```python
from build123d import *

# Parameters (mm, degrees)
F0_W     = 85
F0_H     = 19.05
F0_R     = 1.6
F0_R_2   = 4.75
F1_DEPTH = 6.35
F2_R     = 1.5
F3_DEPTH = 5
F4_R     = 3


with BuildPart() as f1:
    # F0 (on Front) → F1 (new body)
    with BuildSketch(Plane.XZ):
        Rectangle(F0_W, F0_H)
        with Locations((-15.5, 0)):
            Circle(F0_R, mode=Mode.SUBTRACT)
        with Locations((32.5, 0)):
            Circle(F0_R_2, mode=Mode.SUBTRACT)
    extrude(amount=F1_DEPTH)

    # F2 (on face) → F3 (cut)
    with BuildSketch(Plane(origin=(0, 0, -9.525), x_dir=(1, 0, 0), z_dir=(0, 0, -1))):
        with Locations((-25.5, 3.175)):
            Circle(F2_R)
        with Locations((25.5, 3.175)):
            Circle(F2_R)
    extrude(amount=-F3_DEPTH, mode=Mode.SUBTRACT)

    # F4
    f4_edges = [f1.edges().sort_by_distance(p)[0] for p in [
        (-42.5, -3.175, -9.525),
        (42.5, -3.175, -9.525),
        (42.5, -3.175, 9.525),
        (-42.5, -3.175, 9.525),
    ]]
    fillet(f4_edges, radius=F4_R)


solid = f1.part
```
The listing builds one solid part. Answer for the finished solid, in the listing's coordinates (mm). A direction names the side the tool comes from. Give positions to 0.01 mm unless a question says otherwise; leave off trailing zeros. Order: outer loops, then holes, each group sorted by start corner. A loop starts at its lowest first (then second) coordinate and runs counter-clockwise, first axis right, second up.
Item 1: The part is cut by section C-C, the plane y = -5.5. Give the vertices of the cut face in (x, z) (3 decimals).
From the geometry:
outline: (-42.5, -6.525) arc R3 ccw to (-39.5, -9.525) - (39.5, -9.525) arc R3 ccw to (42.5, -6.525) - (42.5, 6.525) arc R3 ccw to (39.5, 9.525) - (-39.5, 9.525) arc R3 ccw to (-42.5, 6.525) - close; hole circle Ø3.2 at (-15.5, 0); hole circle Ø9.5 at (32.5, 0)
Item 2: Given pin 1 Ø2 at (x, z) = (-9, 2.5) entering from +Y; pin 2 Ø0.9 at (x, y) = (25, -4) entering from -Z (3 decimals); pin 3 Ø5.5 at (x, z) = (32.5, 0) entering from -Y, each flat-ended and moving along its own axis, determine where each tip first touches the part or whether it passes through.
From the geometry:
pin 1: stops at y = 0
pin 2: stops at z = -4.525
pin 3: passes through
Item 3: For a pull along Y with two mould halves and no side action, classify faces 3 (the face through (-1, 0, 0)), 4 (the face through (42.5, -3, 0)), 5 (the face through (-26, -3, -4.525)) as pulls with the +Y half, pulls with the -Y half, needs draft (parallel to the pull), parting line crosses it, or undercut.
From the geometry:
face 3: pulls with the +Y half
face 4: needs draft
face 5: undercut
Item 4: The part is cut by section A-A, the plane x = 32.5. Give the vertices of the cut face in (y, z) (3 decimals).
From the geometry:
outline: (-6.35, -9.525) - (0, -9.525) - (0, -4.75) - (-6.35, -4.75) - close; (-6.35, 4.75) - (0, 4.75) - (0, 9.525) - (-6.35, 9.525) - close
Item 5: The part is cut by section D-D, the plane x = -15.5. Give the vertices of the cut face in (y, z) (3 decimals).
From the geometry:
outline: (-6.35, -9.525) - (0, -9.525) - (0, -1.6) - (-6.35, -1.6) - close; (-6.35, 1.6) - (0, 1.6) - (0, 9.525) - (-6.35, 9.525) - close
Item 6: Find the intervals of material crossed by probe 1 along Y at (x, z) = (-25.5, -8.25) (3 decimals); probe 2 along Z at (x, y) = (32.5, -4.5) (3 decimals); probe 3 along X at (y, z) = (-3.25, -7.5), in increasing order.
From the geometry:
probe 1: y = -6.35 to -4.675, -1.675 to 0
probe 2: z = -9.525 to -4.75, 4.75 to 9.525
probe 3: x = -42.34 to -27, -24 to 24, 27 to 42.34
Item 7: The part is cut by section B-B, the plane z = 0. Give the vertices of the cut face in (x, y), and give its area (3 significant figures).
From the geometry:
outline: (-42.5, -6.35) - (-17.1, -6.35) - (-17.1, 0) - (-42.5, 0) - close; (-13.9, -6.35) - (27.75, -6.35) - (27.75, 0) - (-13.9, 0) - close; (37.25, -6.35) - (42.5, -6.35) - (42.5, 0) - (37.25, 0) - close
area: 459 mm2
Item 8: Which of the six approach directions +Z, -Z, +X, -X, +Y, -Y give full straight-line access (tool end or side, diameter ignored) to faces 1 (the face through (-17.1, -3.13, 0.07)), 2 (the face through (25, -3, -4.525))?
From the geometry:
face 1: +Y, -Y
face 2: -Z
